Design review of the part built by this model. Coordinates are the model's own, in mm. Coordinates: 2 decimals unless noted, no trailing zeros. Write each loop counter-clockwise with the first axis right and the second up, starting at its lowest first coordinate (ties: lowest second). Pieces come first, ordered by that corner, then holes. Notation, with made-up numbers: (58.25, -19.5) - (62.25, -19.5) arc R18 ccw to (62.25, -15.5) - close; hole circle Ø8 at (74, 42). An arc over 180 degrees is marked (long way). Use a Markdown table: item, result.
from build123d import *

# Parameters (mm, degrees)
SKETCH1_R           = 43.5
SKETCH1_R_2         = 1.45
BOSS_EXTRUDE1_DEPTH = 3.175
FILLET1_R           = 4
FILLET2_R           = 3.5
SKETCH3_R           = 3.225
BOSS_EXTRUDE2_DEPTH = 3.175


with BuildPart() as part:
    # Sketch1 → Boss-Extrude1 (new body)
    with BuildSketch(Plane.XY):
        Circle(SKETCH1_R)
        with Locations((0, 8)):
            Circle(SKETCH1_R_2, mode=Mode.SUBTRACT)
        with Locations((0, -8)):
            Circle(SKETCH1_R_2, mode=Mode.SUBTRACT)
        with Locations((8, 0)):
            Circle(SKETCH1_R_2, mode=Mode.SUBTRACT)
        with Locations((-8, 0)):
            Circle(SKETCH1_R_2, mode=Mode.SUBTRACT)
        with BuildLine():
            Line((-37.546770833, -2), (-11.882865816, -2))
            ThreePointArc((-11.882865816, -2), (-8.520636713, -8.520636713), (-2, -11.882865816))
            Line((-2, -11.882865816), (-2, -37.546770833))
            ThreePointArc((-2, -37.546770833), (-26.587214973, -26.587214973), (-37.546770833, -2))
        make_face(mode=Mode.SUBTRACT)
        with BuildLine():
            Line((-2, 37.546770833), (-2, 11.882865816))
            ThreePointArc((-2, 11.882865816), (-8.520636713, 8.520636713), (-11.882865816, 2))
            Line((-11.882865816, 2), (-37.546770833, 2))
            ThreePointArc((-37.546770833, 2), (-26.587214973, 26.587214973), (-2, 37.546770833))
        make_face(mode=Mode.SUBTRACT)
        with BuildLine():
            Line((2, 37.546770833), (2, 11.882865816))
            ThreePointArc((2, 11.882865816), (8.520636713, 8.520636713), (11.882865816, 2))
            Line((11.882865816, 2), (37.546770833, 2))
            ThreePointArc((37.546770833, 2), (26.587214973, 26.587214973), (2, 37.546770833))
        make_face(mode=Mode.SUBTRACT)
        with BuildLine():
            Line((11.882865816, -2), (37.546770833, -2))
            ThreePointArc((37.546770833, -2), (26.587214973, -26.587214973), (2, -37.546770833))
            Line((2, -37.546770833), (2, -11.882865816))
            ThreePointArc((2, -11.882865816), (8.520636713, -8.520636713), (11.882865816, -2))
        make_face(mode=Mode.SUBTRACT)
    extrude(amount=BOSS_EXTRUDE1_DEPTH)

    # Fillet1
    fillet1_edges = [part.edges().sort_by_distance(p)[0] for p in [
        (-11.882865816, 2, 1.5875),
        (-2, 11.882865816, 1.5875),
        (-2, -11.882865816, 1.5875),
        (-11.882865816, -2, 1.5875),
        (11.882865816, -2, 1.5875),
        (2, -11.882865816, 1.5875),
        (2, 11.882865816, 1.5875),
        (11.882865816, 2, 1.5875),
    ]]
    fillet(fillet1_edges, radius=FILLET1_R)

    # Fillet2
    fillet2_edges = [part.edges().sort_by_distance(p)[0] for p in [
        (-2, 37.546770833, 1.5875),
        (-37.546770833, 2, 1.5875),
        (-37.546770833, -2, 1.5875),
        (-2, -37.546770833, 1.5875),
        (2, -37.546770833, 1.5875),
        (37.546770833, -2, 1.5875),
        (37.546770833, 2, 1.5875),
        (2, 37.546770833, 1.5875),
    ]]
    fillet(fillet2_edges, radius=FILLET2_R)

    # Sketch3 → Boss-Extrude2 (add)
    with BuildSketch(Plane(origin=(0, 0, 0), x_dir=(-1, 0, 0), z_dir=(0, 0, -1))):
        with Locations(Location((0, 0, 0), (0, 0, 180))):
            Circle(SKETCH3_R)
    extrude(amount=BOSS_EXTRUDE2_DEPTH)


solid = part.part
(1) For pin 1 (1.6 mm diameter, centred on y = -21.5, z = 1, fed in from -X); pin 2 (2.5 mm diameter, centred on y = 28.5, z = 2, fed in from -X); pin 3 (5 mm diameter, centred on x = -8.5, y = 32.5, fed in from +Z); pin 4 (1 mm diameter, centred on y = -1.5, z = -2, fed in from +X), all flat-tipped, find the tip position at first contact; note any pin that passes through.
Determined:
| item | result |
|---|---|
| pin 1 | x = -38.26 |
| pin 2 | x = -33.91 |
| pin 3 | through |
| pin 4 | x = 3.07 |
(2) Take a section at C-C on z = 1.25. State how many separate pieces and enclosed holes the cut face has, and give its area (3 significant figures).
Determined:
| item | result |
|---|---|
| separate pieces | 1 |
| enclosed holes | 8 |
| area | 2,380 mm2 |
(3) Take a section at D-D on y = -31. Write out the cut boundary in (x, z) (3 decimals), and give its area (3 significant figures).
Determined:
| item | result |
|---|---|
| outline | (-30.516, 0) - (-21.278, 0) - (-21.278, 3.175) - (-30.516, 3.175) - close; (-2, 0) - (2, 0) - (2, 3.175) - (-2, 3.175) - close; (21.278, 0) - (30.516, 0) - (30.516, 3.175) - (21.278, 3.175) - close |
| area | 71.4 mm2 |
(4) Take a section at A-A on x = 0. Write out the cut boundary in (y, z) (3 decimals), and give its area (3 significant figures).
Determined:
| item | result |
|---|---|
| outline | (-43.5, 0) - (-9.45, 0) - (-9.45, 3.175) - (-43.5, 3.175) - close; (-6.55, 0) - (-3.225, 0) - (-3.225, -3.175) - (3.225, -3.175) - (3.225, 0) - (6.55, 0) - (6.55, 3.175) - (-6.55, 3.175) - close; (9.45, 0) - (43.5, 0) - (43.5, 3.175) - (9.45, 3.175) - close |
| area | 278 mm2 |
(5) For L1, parallel to Y at x = 0, z = 1.85; L2, parallel to Y at x = -8, z = 0.95; L3, parallel to Y at x = 29.5, z = 1, list the stretches that pass through material, from the lowest coordinate up. Write a range as from..to.
Determined:
| item | result |
|---|---|
| L1 | -43.5..-9.45, -6.55..6.55, 9.45..43.5 |
| L2 | -42.76..-36.74, -9.01..-1.45, 1.45..9.01, 36.74..42.76 |
| L3 | -31.97..-23.31, -2..2, 23.31..31.97 |
(6) Draft analysis for pull direction Y (two halves, no side actions). For faces 1 (the cylindrical face through (-5.66, 43.13, 1.57)), 2 (the cylindrical face through (12.621, 2.704, 1.61)), 3 (the flat face through (-24, 2, 2)), state which applies: +Y half, -Y half, draft (parallel to the pull), parting line (faces both ways), or undercut.
Determined:
| item | result |
|---|---|
| face 1 | parting line |
| face 2 | undercut |
| face 3 | undercut |
